Verification items for the finished model (mm, model axes). Face numbers are marked on the shaded views. A direction names the side the tool comes from. Give positions to 0.01 mm unless a question says otherwise; leave off trailing zeros. Order: outer loops, then holes, each group sorted by start corner. A loop starts at its lowest first (then second) coordinate and runs counter-clockwise, first axis right, second up. Notation, with made-up numbers: (43, 52) -> (50, 52) arc R24 cw to (50, 80) -> close; hole circle Ø5 at (-31.75, 37.25). An arc over 180 degrees is marked (long way). Return JSON: item names as keys, results as strings. Group by question number.
(1) Thickness scan on line 1 along Y through (x, z) = (0, 28.25); line 2 along Y through (x, z) = (0.5, 21); line 3 along Z through (x, y) = (7, -1). Record the ranges inside material, lowest first.
(2) Cross-section at B-B on x = -2. Enter the section's corners in (y, z).
(3) Cross-section at D-D on x = -17.5. Enter the section's corners in (y, z), then the cut area to 3 significant figures.
(4) Cross-section at C-C on z = 20.25. Enter the section's corners in (x, y).
(5) Tool access check on the marked faces 1, 2 and 3. Record the directions out of +Z, -Z, +X, -X, +Y, -Y that give a thin tool (end or side, any length) a straight path to the whole face; none if there is none.
(6) Depth check by flat-ended pin: pin 1 Ø10 at (x, z) = (-9, 18) entering from -Y; pin 2 Ø6 at (x, y) = (0, 0) entering from +Z; pin 3 Ø1 at (x, z) = (10, 18.5) entering from -Y; pin 4 Ø17.5 at (x, y) = (0, 0) entering from -Z. Enter the tip coordinate at first touch or a pass-through.
(7) Release check for a two-part mould opening along Y. For the marked faces 4, 5, 6 and 7 record: pulls with the +Y half, pulls with the -Y half, needs draft (parallel to the pull), parting line crosses it, or undercut.
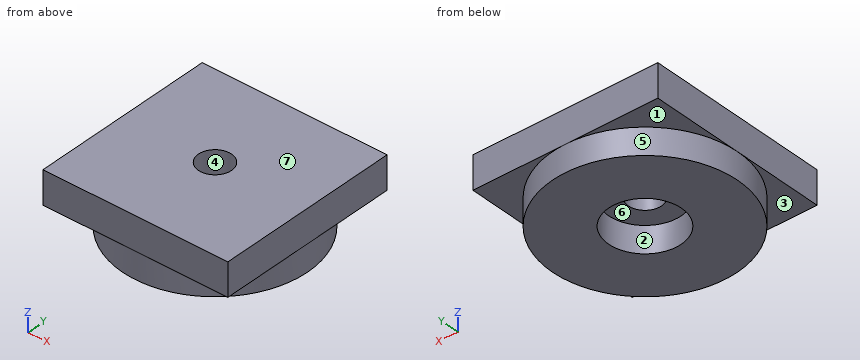
from build123d import *

# Parameters (mm, degrees)
SKETCH1_R           = 28
SKETCH1_R_2         = 18
BOSS_EXTRUDE1_DEPTH = 22
SKETCH2_W           = 56
SKETCH2_H           = 56
BOSS_EXTRUDE2_DEPTH = 10
SKETCH3_W           = 56
SKETCH3_H           = 60.095758966
CUT_EXTRUDE1_DEPTH  = 14
SKETCH4_R           = 5
CUT_EXTRUDE2_DEPTH  = 14
SKETCH5_R           = 21.225012464
SKETCH5_R_2         = 11
BOSS_EXTRUDE3_DEPTH = 8


with BuildPart() as part:
    # Sketch1 → Boss-Extrude1 (new body)
    with BuildSketch(Plane.XY):
        Circle(SKETCH1_R)
        Circle(SKETCH1_R_2, mode=Mode.SUBTRACT)
    extrude(amount=BOSS_EXTRUDE1_DEPTH)

    # Sketch2 → Boss-Extrude2 (add)
    with BuildSketch(Plane.XY.offset(22)):
        Rectangle(SKETCH2_W, SKETCH2_H)
    extrude(amount=BOSS_EXTRUDE2_DEPTH)

    # Sketch3 → Cut-Extrude1 (cut)
    with BuildSketch(Plane(origin=(0, 0, 0), x_dir=(-1, 0, 0), z_dir=(0, 0, -1))):
        with Locations((0, 2.047879483)):
            Rectangle(SKETCH3_W, SKETCH3_H)
    extrude(amount=-CUT_EXTRUDE1_DEPTH, mode=Mode.SUBTRACT)

    # Sketch4 → Cut-Extrude2 (cut)
    with BuildSketch(Plane(origin=(0, 0, 22), x_dir=(-1, 0, 0), z_dir=(0, 0, -1))):
        Circle(SKETCH4_R)
    extrude(amount=-CUT_EXTRUDE2_DEPTH, mode=Mode.SUBTRACT)

    # Sketch5 → Boss-Extrude3 (add)
    with BuildSketch(Plane(origin=(0, 0, 22), x_dir=(-1, 0, 0), z_dir=(0, 0, -1))):
        Circle(SKETCH5_R)
        Circle(SKETCH5_R_2, mode=Mode.SUBTRACT)
    extrude(amount=BOSS_EXTRUDE3_DEPTH)


solid = part.part
Verdict:
{
 "1": {"line 1": "-28 to -5, 5 to 28", "line 2": "-28 to -10.99, 10.99 to 28", "line 3": "22 to 32"},
 "2": {"outline": "(-28, 22) -> (-27.93, 22) -> (-27.93, 14) -> (-10.82, 14) -> (-10.82, 22) -> (-4.58, 22) -> (-4.58, 32) -> (-28, 32) -> close; (4.58, 22) -> (10.82, 22) -> (10.82, 14) -> (27.93, 14) -> (27.93, 22) -> (28, 22) -> (28, 32) -> (4.58, 32) -> close"},
 "3": {"outline": "(-28, 22) -> (-21.86, 22) -> (-21.86, 14) -> (21.86, 14) -> (21.86, 22) -> (28, 22) -> (28, 32) -> (-28, 32) -> close", "area": "910 mm²"},
 "4": {"outline": "circle Ø56 at (0, 0); hole circle Ø22 at (0, 0)"},
 "5": {"face 1": "-Z, -X, +Y", "face 2": "-Z", "face 3": "-Z, -X, -Y"},
 "6": {"pin 1": "y = -28", "pin 2": "through", "pin 3": "y = -26.34", "pin 4": "z = 22"},
 "7": {"face 4": "undercut", "face 5": "parting line crosses it", "face 6": "undercut", "face 7": "needs draft"}
}
